from build123d import *

# Parameters (mm, degrees)
SKETCH1_R                                    = 19.05
SKETCH1_R_2                                  = 17.4244
BOSS_EXTRUDE1_DEPTH                          = 555
CSK_FOR_M2_COUNTERSUNK_FLAT_HEAD_SCR_2_COUNT = 2
CSK_FOR_M2_COUNTERSUNK_FLAT_HEAD_SCR_2_PITCH = 545
CIRPATTERN2_COUNT                            = 2


with BuildPart() as part:
    # Sketch1 → Boss-Extrude1 (new body)
    with BuildSketch(Plane(origin=(0, 0, 0), x_dir=(1, 0, 0), z_dir=(0, 1, 0))):
        with Locations(Location((0, 0, 0), (0, 0, 270))):
            Circle(SKETCH1_R)
        with Locations(Location((0, 0, 0), (0, 0, 270))):
            Circle(SKETCH1_R_2, mode=Mode.SUBTRACT)
    extrude(amount=BOSS_EXTRUDE1_DEPTH)

    # Sketch44 → CSK for M2 Countersunk Flat Head Screw10 (revolve, cut)
    with BuildSketch(Plane(origin=(19.05, 5, 0), x_dir=(0, 0, -1), z_dir=(0, 1, 0))):
        Polygon((0, 0), (0, 10.721032743), (1.2, 10), (1.2, 1), (2.2, 0), align=None)
    csk_for_m2_countersunk_flat_head_screw10 = revolve(axis=Axis((25.4, 5, 0), (-1, 0, 0)), mode=Mode.SUBTRACT)

    # CSK for M2 Countersunk Flat Head Scr 2: CSK for M2 Countersunk Flat Head Screw10 ×2
    with Locations(*[(0, i * CSK_FOR_M2_COUNTERSUNK_FLAT_HEAD_SCR_2_PITCH, 0) for i in range(1, CSK_FOR_M2_COUNTERSUNK_FLAT_HEAD_SCR_2_COUNT)]):
        add(csk_for_m2_countersunk_flat_head_screw10, mode=Mode.SUBTRACT)

    # CirPattern2: CSK for M2 Countersunk Flat Head Screw10 ×2 about axis
    cirpattern2_axis = Axis((0, 555, 0), (0, 1, 0))
    for i in range(1, CIRPATTERN2_COUNT):
        add(csk_for_m2_countersunk_flat_head_screw10.rotate(cirpattern2_axis, i * 360 / CIRPATTERN2_COUNT), mode=Mode.SUBTRACT)

    # CirPattern2 copy 1 sketch → CirPattern2 copy 1 (revolve, cut)
    with BuildSketch(Plane(origin=(-19.05, 550, 0), x_dir=(0, 0, 1), z_dir=(0, 1, 0))):
        Polygon((0, 0), (0, 10.721032743), (1.2, 10), (1.2, 1), (2.2, 0), align=None)
    revolve(axis=Axis((-25.4, 550, 0), (1, 0, 0)), mode=Mode.SUBTRACT)


solid = part.part
Source: CAD feature listing. Evaluate the final solid. Frame: model axes, mm. Give positions to 0.01 mm unless a question says otherwise; leave off trailing zeros. Order: outer loops, then holes, each group sorted by start corner. A loop starts at its lowest first (then second) coordinate and runs counter-clockwise, first axis right, second up. Notation, with made-up numbers: (-12, 16.25) -> (21, 16.25) arc R9 cw to (21, 33.25) -> close; hole circle Ø6 at (8, 75.5). An arc over 180 degrees is marked (long way). Write item = value, one per line.
Q1. Material intervals for line 1 (Y direction, x = -17.65, z = 0); line 2 (Z direction, x = 2, y = 395); line 3 (X direction, y = 456.5, z = -1), sorted ascending. Write a range as from..to.
Data:
line_1 = 0..3.8, 6.2..548.8, 551.2..555
line_2 = -18.94..-17.31, 17.31..18.94
line_3 = -19.02..-17.4, 17.4..19.02
Q2. Cut plane B-B, the plane y = 488. Output: boundary loops of the cut face in (x, z), and give its area (3 significant figures).
Data:
outline = circle Ø38.1 at (0, 0); hole circle Ø34.85 at (0, 0)
area = 186 mm^2
Q3. Cut plane A-A, the plane x = 0. Output: boundary loops of the cut face in (y, z).
Data:
outline = (0, -19.05) -> (555, -19.05) -> (555, -17.42) -> (0, -17.42) -> close; (0, 17.42) -> (555, 17.42) -> (555, 19.05) -> (0, 19.05) -> close
Q4. Pin query (flat end, axial travel): pin 1 (2 mm diameter, centred on y = 5, z = 0, fed in from -X); pin 2 (1 mm diameter, centred on y = 404.5, z = 8.5, fed in from +X); pin 3 (4 mm diameter, centred on y = 163.5, z = 2.5, fed in from +X); pin 4 (3 mm diameter, centred on y = 5, z = 0, fed in from -X). Return the tip coordinate at first contact, or that it passes through.
Data:
pin_1 = through
pin_2 = 17.29
pin_3 = 19.04
pin_4 = -18.35
Q5. Pull-direction query (Z, two-part tool) for faces 1 (the face through (5.23, 273.62, 16.62)), 2 (the face through (-11.59, 273.62, -15.12)), 3 (the face through (-6, 555, 17)); classes: released by +Z, released by -Z, zero draft, split by the parting line, or undercut.
Data:
face_1 = undercut
face_2 = split by the parting line
face_3 = zero draft
